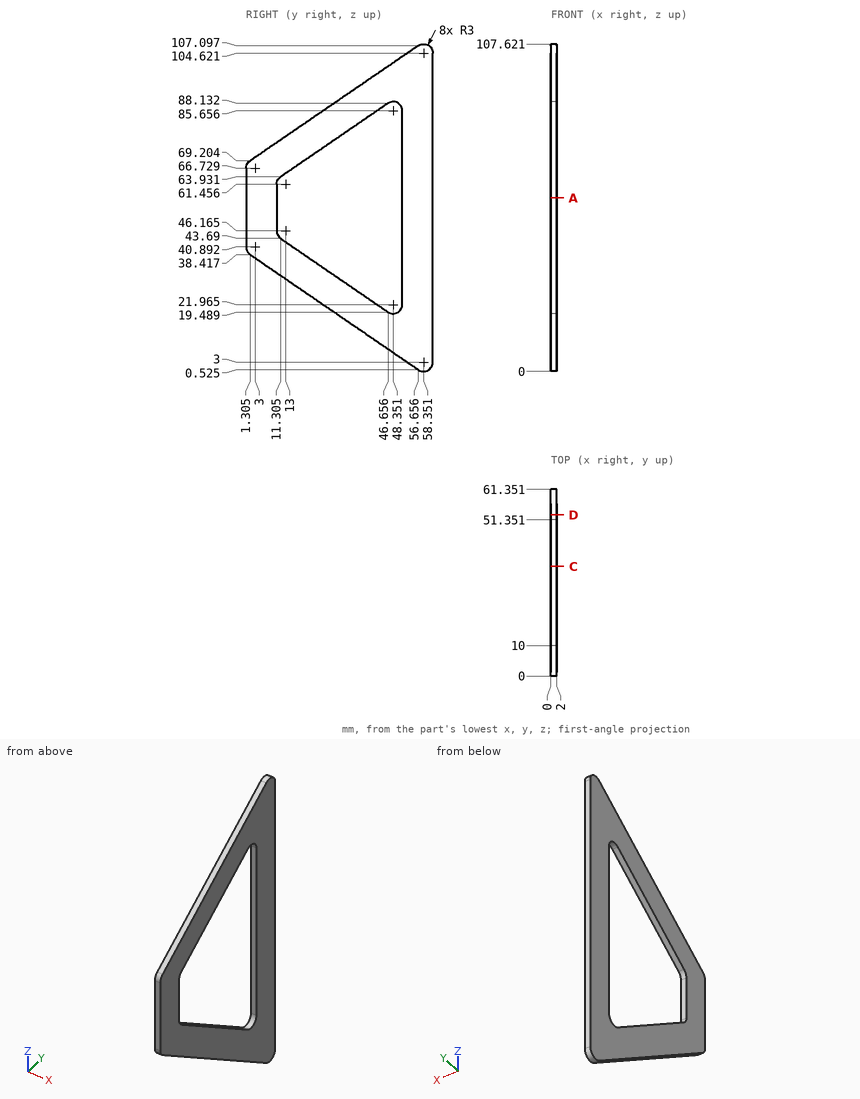
Design review of the part shown in the three views and the two pictorial views. Dimensions are in mm from the part's minimum x, y and z. Give positions to 0.01 mm unless a question says otherwise; leave off trailing zeros. Loops run counter-clockwise (first coordinate to the right, second up) from the corner with the lowest first, then second, coordinate; pieces in that order, holes last. Notation, with made-up numbers: (22, -10) - (27, -10) arc R18 cw to (27, 6) - close; hole circle Ø8 at (25.5, 10.5). An arc over 180 degrees is marked (long way). Write item = value, one per line.
1) Take a section at C-C on y = 36. State the section outline as (x, z) points (1 decimal).
Result sheet:
outline = (0, 14.7) - (2, 14.7) - (2, 26.8) - (0, 26.8) - close; (0, 80.8) - (2, 80.8) - (2, 93) - (0, 93) - close
2) To check wall thickness, follow line 1 (Y direction, x = 0.65, z = 48); line 2 (Z direction, x = 0.3, y = 38) (1 decimal); line 3 (Z direction, x = 0.5, y = 34) (1 decimal). State the ranges of each line that lie inside material, in increasing order.
Result sheet:
line_1 = 0 to 10, 51.35 to 61.35
line_2 = 13.3 to 25.4, 82.2 to 94.3
line_3 = 16 to 28.2, 79.5 to 91.6
3) Take a section at A-A on z = 57. State the section outline as (x, y) points.
Result sheet:
outline = (0, 0) - (2, 0) - (2, 10) - (0, 10) - close; (0, 51.35) - (2, 51.35) - (2, 61.35) - (0, 61.35) - close
4) Clearance check with a flat-ended pin moving along its axis: pin 1 Ø1 at (x, z) = (0.5, 42.5) entering from -Y. State where the tip first meets the part, or that it passes through.
Result sheet:
pin_1 = 0
5) Take a section at D-D on y = 53. State the section outline as (x, z) points, and give its area (3 significant figures).
Result sheet:
outline = (0, 3.03) - (2, 3.03) - (2, 104.59) - (0, 104.59) - close
area = 203 mm2
